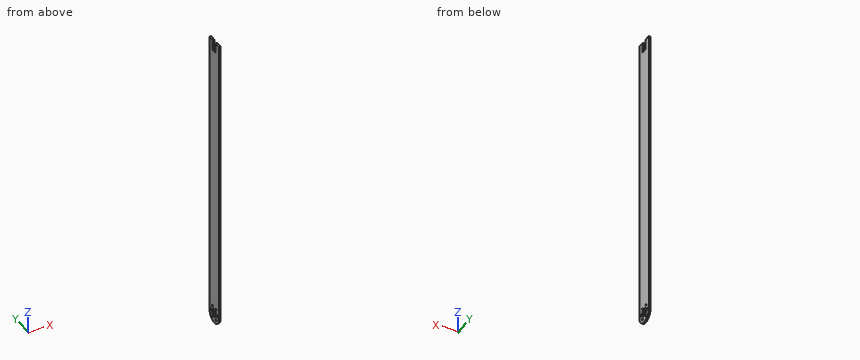
Autodesk Inventor part; units mm, degrees
ref_plane "YZ Plane" through (0, 0, 0) normal (1, 0, 0) x (0, 1, 0)
ref_plane "XZ Plane" through (0, 0, 0) normal (0, 1, 0) x (-1, 0, 0)
ref_plane "XY Plane" through (0, 0, 0) normal (0, 0, 1) x (1, 0, 0)
sketch "Sketch1" plane through (0, 0, 0) normal (1, 0, 0) x (0, 1, 0)
  line L0 (0, -76.2) -> (63.5, -76.2)
  line L1 (63.5, -76.2) -> (63.5, -1193.8)
  line L2 (63.5, -1193.8) -> (0, -1193.8)
  line L3 (0, -1193.8) -> (0, -76.2)
  dimension "d0" = 63.5
  dimension "d1" = 1117.6
extrude "Extrusion1" add sketch "Sketch1" along normal blind 6.35
sketch "Sketch2" plane through (6.35, 0, 0) normal (1, 0, 0) x (0, 0, -1)
  line L0 (1193.8, 63.5) -> (76.2, 63.5)
  line L1 (1155.7, 63.5) -> (1155.7, 0) construction
  line L2 (0, 0) -> (1193.8, 0)
  circle A0 centre (1155.7, 31.75) radius 14.2875
  dimension "d5" = 1155.7
  dimension "d24" = 28.575
extrude "Extrusion2" cut sketch "Sketch2" against normal through all
fillet "Fillet1" radius 31.75 2 edges at (3.175, 63.5, -1193.8) (3.175, 0, -1193.8)
sketch "Sketch5" plane through (6.35, 0, 0) normal (1, 0, 0) x (0, 0, -1)
  circle A0 centre (1155.7, 31.75) radius 14.2875
  line L0 (1155.7, 31.75) -> (1155.7, 55.5752) construction
  circle A1 centre (1155.7, 55.5752) radius 3.6233
  point P0 (0, 0)
  dimension "d32" = 23.8252
extrude "Extrusion5" cut sketch "Sketch5" against normal through all contours A1
pattern_circular "Circular Pattern1" count 6 over 360 about axis through (6.35, 31.75, -1155.7) along (-1, 0, 0) of "Extrusion5"
sketch "Sketch8" plane through (6.35, 0, 0) normal (1, 0, 0) x (0, 0, -1)
  line L0 (76.2, 41.275) -> (114.3, 41.275)
  line L1 (114.3, 41.275) -> (114.3, 22.225)
  line L2 (114.3, 22.225) -> (76.2, 22.225)
  line L3 (76.2, 22.225) -> (76.2, 41.275)
  line L4 (76.2, 63.5) -> (76.2, 0)
  point P0 (0, 0)
  point P1 (76.2, 31.75)
  dimension "d44" = 38.1
  dimension "d45" = 19.05
extrude "Extrusion8" cut sketch "Sketch8" against normal blind 25.4
properties part number "Arm"
CAD build for the part. Positions are in the model's coordinates, mm. Coordinates: 2 decimals unless noted, no trailing zeros. Return JSON: item names as keys, results as strings.
Item 1: Slice it at A-A, the plane x = 2.5. State how many separate pieces and enclosed holes the cut face has, and give its area (3 significant figures).
Findings below:
{"separate pieces": "1", "enclosed holes": "7", "area": "68,900 mm2"}
Item 2: Probe line 1 (Y direction, x = 5.25, z = -1155.7); line 2 (Z direction, x = 5.5, y = 44); line 3 (Z direction, x = 5.5, y = 16.5). List the from-to ranges inside material, lowest first. Write a range as from..to.
Findings below:
{"line 1": "y = 0..4.3, 11.55..17.46, 46.04..51.95, 59.2..63.5", "line 2": "z = -1191.34..-1179.94, -1172.73..-1163.05, -1148.35..-1138.67, -1131.46..-76.2", "line 3": "z = -1189.9..-1177.74, -1174.92..-1136.48, -1133.66..-76.2"}
Item 3: Drop flat-ended pins along their axis: pin 1 Ø3 at (x, y) = (3, 45.5) entering from -Z; pin 2 Ø3 at (x, y) = (2, 35.5) entering from +Z. Give the stop position or say it passes through.
Findings below:
{"pin 1": "stops at z = -1191.34", "pin 2": "stops at z = -114.3"}
